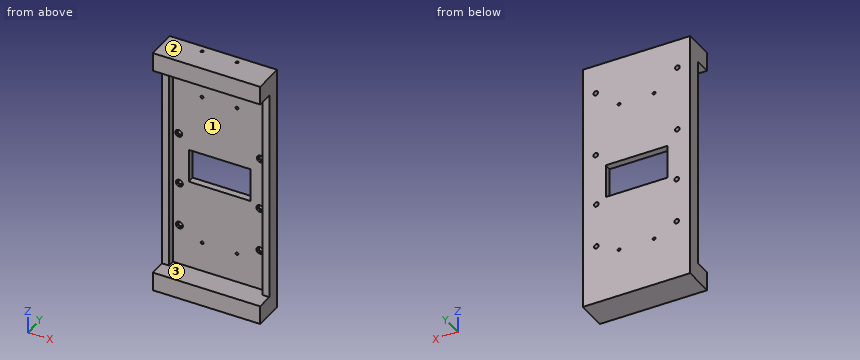
from build123d import *

# Parameters (mm, degrees)
SKETCH_4_W           = 46
SKETCH_4_H           = 107.5
EXTRUDE_1_DEPTH      = 3
SKETCH_5_W           = 23.5
SKETCH_5_H           = 56
EXTRUDE_2_DEPTH      = 12.4
SKETCH_6_R           = 1.75
SKETCH_6_R_2         = 0.75
CUT_EXTRUDE_1_DEPTH  = 66.1949768
SKETCH_6_3_R         = 3
CUT_EXTRUDE_2_DEPTH  = 2.7
CUT_EXTRUDE_START    = -20.8
SKETCH_6_4_R         = 3
CUT_EXTRUDE_3_DEPTH  = 2.7
SKETCH_6_5_R         = 1.5
CUT_EXTRUDE_4_DEPTH  = 1.2
CUT_EXTRUDE_START_2  = -22.3
SKETCH_6_6_R         = 1.5
CUT_EXTRUDE_5_DEPTH  = 1.2
SKETCH_7_R           = 0.7
CUT_EXTRUDE_6_DEPTH  = 2
CUT_EXTRUDE_START_3  = -2
SKETCH_8_W           = 16.4
SKETCH_8_H           = 14.4
CUT_EXTRUDE_7_DEPTH  = 59.458436136
SKETCH_9_W           = 46
SKETCH_9_H           = 8
EXTRUDE_3_DEPTH      = 10
SKETCH_9_3_W         = 3
SKETCH_9_3_H         = 91.5
EXTRUDE_4_DEPTH      = 3
SKETCH_10_R          = 0.6
CUT_EXTRUDE_8_DEPTH  = 2
SKETCH_11_W          = 26.4
SKETCH_11_H          = 14.4
CUT_EXTRUDE_9_DEPTH  = 5
SKETCH_12_R          = 0.5
CUT_EXTRUDE_10_DEPTH = 2
CUT_EXTRUDE_11_DEPTH = 61.458436136
SKETCH_15_R          = 0.6
CUT_EXTRUDE_13_DEPTH = 60.764726219
SKETCH_14_W          = 23.5
SKETCH_14_H          = 12.4
CUT_EXTRUDE_12_DEPTH = 56
SKETCH_16_R          = 1
CUT_EXTRUDE_14_DEPTH = 60.313257371
SKETCH_16_3_R        = 1.5
SKETCH_16_3_R_2      = 1
CUT_EXTRUDE_15_DEPTH = 1
SKETCH_17_R          = 1
CUT_EXTRUDE_16_DEPTH = 60.313257371
SKETCH_18_R          = 1.5
CUT_EXTRUDE_17_DEPTH = 1


with BuildPart() as part:
    # 草图4 → 凸台-拉伸1 (new body)
    with BuildSketch(Plane(origin=(0, 0, 0), x_dir=(1, 0, 0), z_dir=(0, 1, 0))):
        Rectangle(SKETCH_4_W, SKETCH_4_H)
    extrude(amount=EXTRUDE_1_DEPTH)

    # 草图5 → 凸台-拉伸2 (add)
    with BuildSketch(Plane.XZ):
        Rectangle(SKETCH_5_W, SKETCH_5_H)
    extrude(amount=EXTRUDE_2_DEPTH)

    # 草图6 → 切除-拉伸1 (cut, through all)
    with BuildSketch(Plane.ZY.offset(11.75)):
        with Locations((0, -12.4)):
            Circle(SKETCH_6_R)
        with Locations((25, -12.4)):
            Circle(SKETCH_6_R_2)
        with Locations((-25, -12.4)):
            Circle(SKETCH_6_R_2)
    extrude(amount=-CUT_EXTRUDE_1_DEPTH, mode=Mode.SUBTRACT)

    # 草图6<3> → 切除-拉伸2 (cut)
    with BuildSketch(Plane.ZY.offset(11.75)):
        with Locations((0, -12.4)):
            Circle(SKETCH_6_3_R)
    extrude(amount=-CUT_EXTRUDE_2_DEPTH, mode=Mode.SUBTRACT)

    # 草图6<4> → 切除-拉伸3 (cut)
    with BuildSketch(Plane.ZY.offset(11.75).offset(CUT_EXTRUDE_START)):
        with Locations((0, -12.4)):
            Circle(SKETCH_6_4_R)
    extrude(amount=-CUT_EXTRUDE_3_DEPTH, mode=Mode.SUBTRACT)

    # 草图6<5> → 切除-拉伸4 (cut)
    with BuildSketch(Plane.ZY.offset(11.75)):
        with Locations((25, -12.4)):
            Circle(SKETCH_6_5_R)
        with Locations((-25, -12.4)):
            Circle(SKETCH_6_5_R)
    extrude(amount=-CUT_EXTRUDE_4_DEPTH, mode=Mode.SUBTRACT)

    # 草图6<6> → 切除-拉伸5 (cut)
    with BuildSketch(Plane.ZY.offset(11.75).offset(CUT_EXTRUDE_START_2)):
        with Locations((25, -12.4)):
            Circle(SKETCH_6_6_R)
        with Locations((-25, -12.4)):
            Circle(SKETCH_6_6_R)
    extrude(amount=-CUT_EXTRUDE_5_DEPTH, mode=Mode.SUBTRACT)

    # 草图7 → 切除-拉伸6 (cut)
    with BuildSketch(Plane(origin=(0, -12.4, 0), x_dir=(-1, 0, 0), z_dir=(0, -1, 0))):
        with Locations(Location((9.249949764, -20, 0), (0, 0, 90))):
            Circle(SKETCH_7_R)
        with Locations(Location((-9.249949764, -20, 0), (0, 0, 90))):
            Circle(SKETCH_7_R)
        with Locations(Location((-9.249949764, -6, 0), (0, 0, 90))):
            Circle(SKETCH_7_R)
        with Locations(Location((9.249949764, -6, 0), (0, 0, 90))):
            Circle(SKETCH_7_R)
        with Locations(Location((9.249949764, 6, 0), (0, 0, 90))):
            Circle(SKETCH_7_R)
        with Locations(Location((-9.249949764, 6, 0), (0, 0, 90))):
            Circle(SKETCH_7_R)
        with Locations(Location((-9.249949764, 20, 0), (0, 0, 90))):
            Circle(SKETCH_7_R)
        with Locations(Location((9.249949764, 20, 0), (0, 0, 90))):
            Circle(SKETCH_7_R)
    extrude(amount=-CUT_EXTRUDE_6_DEPTH, mode=Mode.SUBTRACT)

    # 草图8 → 切除-拉伸7 (cut, through all)
    with BuildSketch(Plane.XZ.offset(12.4).offset(CUT_EXTRUDE_START_3)):
        Rectangle(SKETCH_8_W, SKETCH_8_H)
    extrude(amount=-CUT_EXTRUDE_7_DEPTH, mode=Mode.SUBTRACT)

    # 草图9 → 凸台-拉伸3 (add)
    with BuildSketch(Plane.XZ):
        with Locations((0, 49.75)):
            Rectangle(SKETCH_9_W, SKETCH_9_H)
        with Locations((0, -49.75)):
            Rectangle(SKETCH_9_W, SKETCH_9_H)
    extrude(amount=EXTRUDE_3_DEPTH)

    # 草图9<3> → 凸台-拉伸4 (add)
    with BuildSketch(Plane.XZ):
        with Locations((-21.5, 0)):
            Rectangle(SKETCH_9_3_W, SKETCH_9_3_H)
        with Locations((21.5, 0)):
            Rectangle(SKETCH_9_3_W, SKETCH_9_3_H)
    extrude(amount=EXTRUDE_4_DEPTH)

    # 草图10 → 切除-拉伸8 (cut)
    with BuildSketch(Plane.XY.offset(53.75)):
        with Locations((-7.5, 0)):
            Circle(SKETCH_10_R)
        with Locations((7.5, 0)):
            Circle(SKETCH_10_R)
    extrude(amount=-CUT_EXTRUDE_8_DEPTH, mode=Mode.SUBTRACT)

    # 草图11 → 切除-拉伸9 (cut)
    with BuildSketch(Plane(origin=(0, 3, 0), x_dir=(1, 0, 0), z_dir=(0, 1, 0))):
        Rectangle(SKETCH_11_W, SKETCH_11_H)
    extrude(amount=-CUT_EXTRUDE_9_DEPTH, mode=Mode.SUBTRACT)

    # 草图12 → 切除-拉伸10 (cut)
    with BuildSketch(Plane(origin=(0, -2, 0), x_dir=(1, 0, 0), z_dir=(0, 1, 0))):
        with Locations(Location((-9.975, 0, 0), (0, 0, 270))):
            Circle(SKETCH_12_R)
        with Locations(Location((9.975, 0, 0), (0, 0, 270))):
            Circle(SKETCH_12_R)
    extrude(amount=-CUT_EXTRUDE_10_DEPTH, mode=Mode.SUBTRACT)

    # 草图13 → 切除-拉伸11 (cut, through all)
    with BuildSketch(Plane.XZ.offset(12.4)):
        Polygon((-8.75, 2.6), (-6.75, 2.6), (-6.75, 5.75), (-3.55, 5.75), (-3.55, -5.75), (-6.75, -5.75), (-6.75, -2.6), (-8.75, -2.6), align=None)
    extrude(amount=-CUT_EXTRUDE_11_DEPTH, mode=Mode.SUBTRACT)

    # 草图15 → 切除-拉伸13 (cut, through all)
    with BuildSketch(Plane.XZ):
        with Locations(Location((-7.5, 33, 0), (0, 0, 270))):
            Circle(SKETCH_15_R)
        with Locations(Location((7.5, 33, 0), (0, 0, 270))):
            Circle(SKETCH_15_R)
        with Locations(Location((-7.5, -33, 0), (0, 0, 270))):
            Circle(SKETCH_15_R)
        with Locations(Location((7.5, -33, 0), (0, 0, 270))):
            Circle(SKETCH_15_R)
    extrude(amount=-CUT_EXTRUDE_13_DEPTH, mode=Mode.SUBTRACT)

    # 草图14 → 切除-拉伸12 (cut)
    with BuildSketch(Plane(origin=(0, 0, -28), x_dir=(-1, 0, 0), z_dir=(0, 0, -1))):
        with Locations((0, -6.2)):
            Rectangle(SKETCH_14_W, SKETCH_14_H)
    extrude(amount=-CUT_EXTRUDE_12_DEPTH, mode=Mode.SUBTRACT)

    # 草图16 → 切除-拉伸14 (cut, through all)
    with BuildSketch(Plane(origin=(0, 0, 0), x_dir=(-1, 0, 0), z_dir=(0, -1, 0))):
        with Locations(Location((17.25, 9.25, 0), (0, 0, 90))):
            Circle(SKETCH_16_R)
        with Locations(Location((17.25, 28.25, 0), (0, 0, 90))):
            Circle(SKETCH_16_R)
        with Locations(Location((-17.25, 28.25, 0), (0, 0, 90))):
            Circle(SKETCH_16_R)
        with Locations(Location((-17.25, 9.25, 0), (0, 0, 90))):
            Circle(SKETCH_16_R)
    extrude(amount=-CUT_EXTRUDE_14_DEPTH, mode=Mode.SUBTRACT)

    # 草图16<3> → 切除-拉伸15 (cut)
    # profile 1 of 4: a face of its own
    with BuildSketch(Plane(origin=(0, 0, 0), x_dir=(-1, 0, 0), z_dir=(0, -1, 0))):
        with Locations(Location((-17.25, 28.25, 0), (0, 0, 90))):
            Circle(SKETCH_16_3_R)
        with Locations(Location((-17.25, 28.25, 0), (0, 0, 90))):
            Circle(SKETCH_16_3_R_2, mode=Mode.SUBTRACT)
    # profile 2 of 4: a face of its own
    with BuildSketch(Plane(origin=(0, 0, 0), x_dir=(-1, 0, 0), z_dir=(0, -1, 0))):
        with Locations(Location((-17.25, 9.25, 0), (0, 0, 90))):
            Circle(SKETCH_16_3_R)
        with Locations(Location((-17.25, 9.25, 0), (0, 0, 90))):
            Circle(SKETCH_16_3_R_2, mode=Mode.SUBTRACT)
    # profile 3 of 4: a face of its own
    with BuildSketch(Plane(origin=(0, 0, 0), x_dir=(-1, 0, 0), z_dir=(0, -1, 0))):
        with Locations(Location((17.25, 9.25, 0), (0, 0, 90))):
            Circle(SKETCH_16_3_R)
        with Locations(Location((17.25, 9.25, 0), (0, 0, 90))):
            Circle(SKETCH_16_3_R_2, mode=Mode.SUBTRACT)
    # profile 4 of 4: a face of its own
    with BuildSketch(Plane(origin=(0, 0, 0), x_dir=(-1, 0, 0), z_dir=(0, -1, 0))):
        with Locations(Location((17.25, 28.25, 0), (0, 0, 90))):
            Circle(SKETCH_16_3_R)
        with Locations(Location((17.25, 28.25, 0), (0, 0, 90))):
            Circle(SKETCH_16_3_R_2, mode=Mode.SUBTRACT)
    extrude(amount=-CUT_EXTRUDE_15_DEPTH, mode=Mode.SUBTRACT)

    # 草图17 → 切除-拉伸16 (cut, through all)
    with BuildSketch(Plane.XZ):
        with Locations(Location((17.5, 41.25, 0), (0, 0, 270))):
            Circle(SKETCH_17_R)
        with Locations(Location((17.5, 13.25, 0), (0, 0, 270))):
            Circle(SKETCH_17_R)
        with Locations(Location((-17.5, 13.25, 0), (0, 0, 270))):
            Circle(SKETCH_17_R)
        with Locations(Location((-17.5, 41.25, 0), (0, 0, 270))):
            Circle(SKETCH_17_R)
    extrude(amount=-CUT_EXTRUDE_16_DEPTH, mode=Mode.SUBTRACT)

    # 草图18 → 切除-拉伸17 (cut)
    with BuildSketch(Plane.XZ):
        with Locations(Location((-17.5, 13.25, 0), (0, 0, 270))):
            Circle(SKETCH_18_R)
        with Locations(Location((17.5, 13.25, 0), (0, 0, 270))):
            Circle(SKETCH_18_R)
        with Locations(Location((17.5, 41.25, 0), (0, 0, 270))):
            Circle(SKETCH_18_R)
        with Locations(Location((-17.5, 41.25, 0), (0, 0, 270))):
            Circle(SKETCH_18_R)
    extrude(amount=-CUT_EXTRUDE_17_DEPTH, mode=Mode.SUBTRACT)


solid = part.part
Design review of the part built by this model. Coordinates are the model's own, in mm. Face numbers are marked on the shaded views. Coordinates: 2 decimals unless noted, no trailing zeros. Loops run counter-clockwise (first coordinate to the right, second up) from the corner with the lowest first, then second, coordinate; pieces in that order, holes last. Notation, with made-up numbers: (7.25, 2) - (25.25, 2) arc R15 ccw to (25.25, 22) - close; hole circle Ø9 at (67, 48.5). An arc over 180 degrees is marked (long way). Use CSV: the item, a comma, the result in double quotes. Start each with the question number.
1. Add section B-B on z = 13.25. Give the boundary of the cut face in (x, y), plus the area to 3 significant figures.
2. Add section A-A on y = -7.25. Give the boundary of the cut face in (x, z), plus the area to 3 significant figures.
3. Clearance check with flat-ended pins moving along their axes: pin 1 (2.5 mm diameter, centred on x = 17.5, z = 13.25, fed in from -Y); pin 2 (2.5 mm diameter, centred on x = -16.5, z = -28.5, fed in from -Y). State where each tip first meets the part, or that it passes through.
4. To check wall thickness, follow probe 1 along X at (y, z) = (2.4, 41.25); probe 2 along X at (y, z) = (1.4, -28.25); probe 3 along Z at (x, y) = (-19.5, -7.5). State the ranges of each line that lie inside material, in increasing order.
5. Add section C-C on x = 3. Give the boundary of the cut face in (y, z), plus the area to 3 significant figures.
6. Mouldability with a two-part tool opening along X and no side actions: class the marked faces 1, 2 and 3 as released by +X, released by -X, zero draft, split by the parting line, or undercut.
7. Add section D-D on y = -2. Give the boundary of the cut face in (x, z), plus the area to 4 significant figures.
Resolved:
1,outline,"(-23, -3) - (-20, -3) - (-20, 0) - (-19, 0) - (-19, 1) - (-18.5, 1) - (-18.5, 3) - (-23, 3) - close; (-16.5, 1) - (-16, 1) - (-16, 0) - (16, 0) - (16, 1) - (16.5, 1) - (16.5, 3) - (-16.5, 3) - close; (18.5, 1) - (19, 1) - (19, 0) - (20, 0) - (20, -3) - (23, -3) - (23, 3) - (18.5, 3) - close"
1,area,"142 mm2"
2,outline,"(-23, -53.75) - (23, -53.75) - (23, -45.75) - (-23, -45.75) - close; (-23, 45.75) - (23, 45.75) - (23, 53.75) - (-23, 53.75) - close"
2,area,"736 mm2"
3,pin 1,"y = 1"
3,pin 2,"y = 0"
4,probe 1,"-23 to -18.5, -16.5 to 16.5, 18.5 to 23"
4,probe 2,"-23 to -18.25, -16.25 to 16.25, 18.25 to 23"
4,probe 3,"-53.75 to -45.75, 45.75 to 53.75"
5,outline,"(-10, -53.75) - (3, -53.75) - (3, -7.2) - (0, -7.2) - (0, -45.75) - (-10, -45.75) - close; (-10, 45.75) - (0, 45.75) - (0, 7.2) - (3, 7.2) - (3, 53.75) - (-10, 53.75) - close"
5,area,"439 mm2"
6,face 1,"undercut"
6,face 2,"zero draft"
6,face 3,"undercut"
7,outline,"(-23, -53.75) - (23, -53.75) - (23, 53.75) - (-23, 53.75) - close; hole (-20, -45.75) - (20, -45.75) - (20, 45.75) - (-20, 45.75) - close"
7,area,"1,285 mm2"
